Geometry check sheet. Reference: drawing and pictorial views, mm from the part's lowest x, y, z. A direction names the side the tool comes from. Give positions to 0.01 mm unless a question says otherwise; leave off trailing zeros. Loops run counter-clockwise (first coordinate to the right, second up) from the corner with the lowest first, then second, coordinate; pieces in that order, holes last. Notation, with made-up numbers: (1.5, -5.75) - (38.5, -5.75) arc R6 ccw to (38.5, 4.25) - close; hole circle Ø2 at (15.25, 49.5). An arc over 180 degrees is marked (long way). Use CSV: the item, a comma, the result in double quotes.
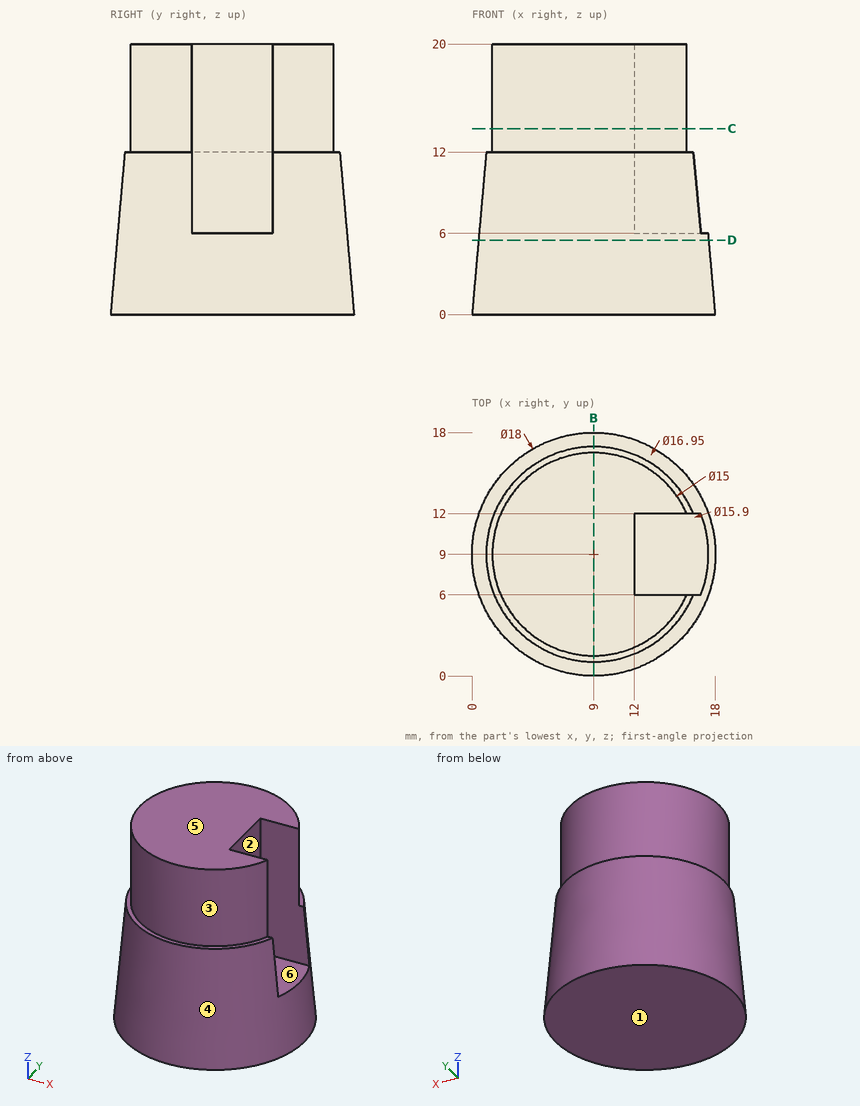
1. Sectioned sample at D-D, the plane z = 5.5. Record the boundary of the cut face in (x, y).
Completed:
outline,"circle Ø17.04 at (9, 9)"
2. Set-up check for the marked faces 1, 2 and 3: record each of +Z, -Z, +X, -X, +Y, -Y from which the full face is reachable in a straight line by a thin tool's end or side.
Completed:
face 1,"-Z, +X, -X, +Y, -Y"
face 2,"+Z, +X"
face 3,"+Z"
3. Scan lines: line 1 along Y through (x, z) = (12.75, 16.5) (1 decimal); line 2 along X through (y, z) = (11.5, 7.5); line 3 along Y through (x, z) = (9.25, 13.5). Record each from-to range of solid material in increasing order.
Completed:
line 1,"y = 2.5 to 6, 12 to 15.5"
line 2,"x = 1.04 to 12"
line 3,"y = 1.5 to 16.5"
4. Release check for a two-part mould opening along Y. For the marked faces 4, 5 and 6 record: released by +Y, released by -Y, zero draft, split by the parting line, or undercut.
Completed:
face 4,"split by the parting line"
face 5,"zero draft"
face 6,"undercut"
5. Go/stop test with flat-tipped pins: pin 1 Ø1.5 at (x, z) = (7.5, 9) entering from +Y; pin 2 Ø2 at (y, z) = (14.5, 17) entering from +X; pin 3 Ø4 at (x, z) = (7.5, 17) entering from -Y. Record where each tip stops, or that it passes through.
Completed:
pin 1,"stops at y = 17.2"
pin 2,"stops at x = 15"
pin 3,"stops at y = 1.5"
6. Sectioned sample at C-C, the plane z = 13.75. Record the boundary of the cut face in (x, y).
Completed:
outline,"(12, 6) - (12, 12) - (15.87, 12) arc R7.5 ccw (long way) to (15.87, 6) - close"
7. Sectioned sample at B-B, the plane x = 9. Record the boundary of the cut face in (y, z).
Completed:
outline,"(0, 0) - (18, 0) - (16.95, 12) - (16.5, 12) - (16.5, 20) - (1.5, 20) - (1.5, 12) - (1.05, 12) - close"
